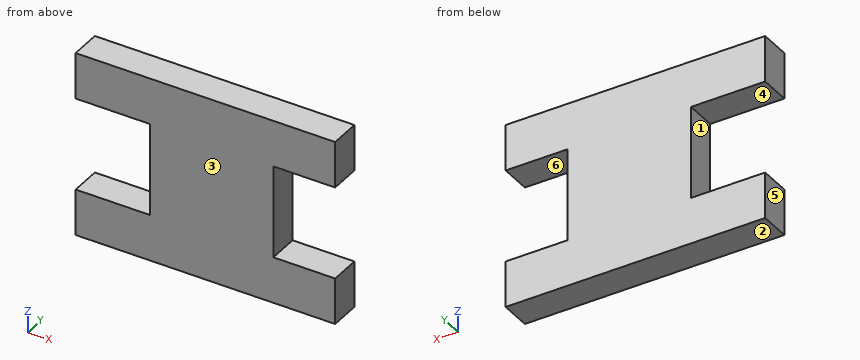
```python
from build123d import *

# Parameters (mm, degrees)
SKETCH1_W           = 95
SKETCH1_H           = 30
SKETCH1_R           = 7
SKETCH1_R_2         = 1
BOSS_EXTRUDE1_DEPTH = 5
SKETCH3_W           = 5
SKETCH3_H           = 10
CUT_EXTRUDE2_DEPTH  = 10
SKETCH4_R           = 7
SKETCH4_R_2         = 1
CUT_EXTRUDE3_DEPTH  = 10
FILLET1_R           = 10
CUT_EXTRUDE4_REACH  = 7
SKETCH5_R           = 2.05
BOSS_EXTRUDE2_DEPTH = 5
CUT_EXTRUDE5_DEPTH  = 5


with BuildPart() as part:
    # Sketch1 → Boss-Extrude1 (new body)
    with BuildSketch(Plane(origin=(0, 0, 0), x_dir=(1, 0, 0), z_dir=(0, 1, 0))):
        Rectangle(SKETCH1_W, SKETCH1_H)
        with Locations((-32.5, 0)):
            Circle(SKETCH1_R, mode=Mode.SUBTRACT)
        with Locations((-42.9, 0)):
            Circle(SKETCH1_R_2, mode=Mode.SUBTRACT)
        with Locations((-45.9, 0)):
            Circle(SKETCH1_R_2, mode=Mode.SUBTRACT)
        with Locations((-32.5, 10.4)):
            Circle(SKETCH1_R_2, mode=Mode.SUBTRACT)
        with Locations((-32.5, 13.4)):
            Circle(SKETCH1_R_2, mode=Mode.SUBTRACT)
        with Locations((-22.1, 0)):
            Circle(SKETCH1_R_2, mode=Mode.SUBTRACT)
        with Locations((-19.1, 0)):
            Circle(SKETCH1_R_2, mode=Mode.SUBTRACT)
        with Locations((-32.5, -10.4)):
            Circle(SKETCH1_R_2, mode=Mode.SUBTRACT)
        with Locations((-32.5, -13.4)):
            Circle(SKETCH1_R_2, mode=Mode.SUBTRACT)
    extrude(amount=BOSS_EXTRUDE1_DEPTH)

    # Sketch3 → Cut-Extrude2 (cut)
    with BuildSketch(Plane(origin=(0, 5, 0), x_dir=(1, 0, 0), z_dir=(0, 1, 0))):
        with Locations((-5, 0)):
            Rectangle(SKETCH3_W, SKETCH3_H)
    extrude(amount=-CUT_EXTRUDE2_DEPTH, mode=Mode.SUBTRACT)

    # Sketch4 → Cut-Extrude3 (cut)
    with BuildSketch(Plane(origin=(0, 5, 0), x_dir=(1, 0, 0), z_dir=(0, 1, 0))):
        with Locations((-32.5, 0)):
            Circle(SKETCH4_R)
        with Locations((-32.5, -13.4)):
            Circle(SKETCH4_R_2)
        with Locations((-32.5, -10.4)):
            Circle(SKETCH4_R_2)
        with Locations((-42.9, 0)):
            Circle(SKETCH4_R_2)
        with Locations((-45.9, 0)):
            Circle(SKETCH4_R_2)
        with Locations((-32.5, 13.4)):
            Circle(SKETCH4_R_2)
        with Locations((-22.1, 0)):
            Circle(SKETCH4_R_2)
        with Locations((-19.1, 0)):
            Circle(SKETCH4_R_2)
        with Locations((-32.5, 10.4)):
            Circle(SKETCH4_R_2)
        with Locations((27.5, -13.4)):
            Circle(SKETCH4_R_2)
        with Locations((27.5, -10.4)):
            Circle(SKETCH4_R_2)
        with Locations((40.9, 0)):
            Circle(SKETCH4_R_2)
        with Locations((37.9, 0)):
            Circle(SKETCH4_R_2)
        with Locations((27.5, 0)):
            Circle(SKETCH4_R)
        with Locations((27.5, 10.4)):
            Circle(SKETCH4_R_2)
        with Locations((27.5, 13.4)):
            Circle(SKETCH4_R_2)
        with Locations((17.1, 0)):
            Circle(SKETCH4_R_2)
        with Locations((14.1, 0)):
            Circle(SKETCH4_R_2)
    extrude(amount=-CUT_EXTRUDE3_DEPTH, mode=Mode.SUBTRACT)

    # Fillet1
    fillet1_edges = [part.edges().sort_by_distance(p)[0] for p in [
        (47.5, 2.5, 15),
        (-47.5, 2.5, 15),
        (-47.5, 2.5, -15),
        (47.5, 2.5, -15),
    ]]
    fillet(fillet1_edges, radius=FILLET1_R)

    # Sketch5 → Cut-Extrude4 (cut, up to next)
    with BuildSketch(Plane(origin=(0, 5, 0), x_dir=(1, 0, 0), z_dir=(0, 1, 0)), mode=Mode.PRIVATE) as cut_extrude4_sk1:
        with Locations((-7.5, 5)):
            Circle(SKETCH5_R)
    cut_extrude4_tool1 = extrude(cut_extrude4_sk1.sketch, amount=-CUT_EXTRUDE4_REACH, mode=Mode.PRIVATE) & part.part
    add(cut_extrude4_tool1.solids().sort_by_distance((-7.5, 5, -5))[0], mode=Mode.SUBTRACT)
    # Sketch5 → Cut-Extrude4 (cut, up to next)
    with BuildSketch(Plane(origin=(0, 5, 0), x_dir=(1, 0, 0), z_dir=(0, 1, 0)), mode=Mode.PRIVATE) as cut_extrude4_sk2:
        with Locations((-2.5, 5)):
            Circle(SKETCH5_R)
    cut_extrude4_tool2 = extrude(cut_extrude4_sk2.sketch, amount=-CUT_EXTRUDE4_REACH, mode=Mode.PRIVATE) & part.part
    add(cut_extrude4_tool2.solids().sort_by_distance((-2.5, 5, -5))[0], mode=Mode.SUBTRACT)
    # Sketch5 → Cut-Extrude4 (cut, up to next)
    with BuildSketch(Plane(origin=(0, 5, 0), x_dir=(1, 0, 0), z_dir=(0, 1, 0)), mode=Mode.PRIVATE) as cut_extrude4_sk3:
        with Locations((-2.5, -5)):
            Circle(SKETCH5_R)
    cut_extrude4_tool3 = extrude(cut_extrude4_sk3.sketch, amount=-CUT_EXTRUDE4_REACH, mode=Mode.PRIVATE) & part.part
    add(cut_extrude4_tool3.solids().sort_by_distance((-2.5, 5, 5))[0], mode=Mode.SUBTRACT)
    # Sketch5 → Cut-Extrude4 (cut, up to next)
    with BuildSketch(Plane(origin=(0, 5, 0), x_dir=(1, 0, 0), z_dir=(0, 1, 0)), mode=Mode.PRIVATE) as cut_extrude4_sk4:
        with Locations((-7.5, -5)):
            Circle(SKETCH5_R)
    cut_extrude4_tool4 = extrude(cut_extrude4_sk4.sketch, amount=-CUT_EXTRUDE4_REACH, mode=Mode.PRIVATE) & part.part
    add(cut_extrude4_tool4.solids().sort_by_distance((-7.5, 5, 5))[0], mode=Mode.SUBTRACT)

    # Sketch6 → Boss-Extrude2 (add)
    with BuildSketch(Plane(origin=(0, 5, 0), x_dir=(1, 0, 0), z_dir=(0, 1, 0))):
        Polygon((-22.5, 15), (19.5, 15), (19.5, 7.5), (9.5, 7.5), (9.5, -7.5), (19.5, -7.5), (19.5, -15), (-22.5, -15), (-22.5, -7.5), (-10.5, -7.5), (-10.5, 7.5), (-22.5, 7.5), align=None)
    extrude(amount=BOSS_EXTRUDE2_DEPTH)

    # Sketch8 → Cut-Extrude5 (cut)
    with BuildSketch(Plane.XZ):
        with BuildLine():
            Line((47.5, -5), (47.5, 5))
            ThreePointArc((47.5, 5), (44.571067812, 12.071067812), (37.5, 15))
            Line((37.5, 15), (-37.5, 15))
            ThreePointArc((-37.5, 15), (-44.571067812, 12.071067812), (-47.5, 5))
            Line((-47.5, 5), (-47.5, -5))
            ThreePointArc((-47.5, -5), (-44.571067812, -12.071067812), (-37.5, -15))
            Line((-37.5, -15), (37.5, -15))
            ThreePointArc((37.5, -15), (44.571067812, -12.071067812), (47.5, -5))
        make_face()
    extrude(amount=-CUT_EXTRUDE5_DEPTH, mode=Mode.SUBTRACT)


solid = part.part
```
Geometry check sheet. Reference: the model listing, model coordinates, mm. Face numbers are marked on the shaded views. A direction names the side the tool comes from. Coordinates: 2 decimals unless noted, no trailing zeros. Order: outer loops, then holes, each group sorted by start corner. A loop starts at its lowest first (then second) coordinate and runs counter-clockwise, first axis right, second up. Notation, with made-up numbers: (60, -11) - (78, -11) arc R19 cw to (78, -5) - close; hole circle Ø5 at (18.5, -29.75). An arc over 180 degrees is marked (long way). Answer as a JSON object with one key per item and string values. Group by question number.
Item 1: Sectioned sample at A-A, the plane x = 14. Record the cut outline in (y, z), and give its area (3 significant figures).
Item 2: Sectioned sample at C-C, the plane z = -6.5. Record the cut outline in (x, y).
Item 3: Draft check along Z on the marked faces 1, 2 and 3. Enter one of: +Z half, -Z half, draft (parallel to the pull), parting line (faces both ways), or undercut.
Item 4: Sectioned sample at B-B, the plane y = 7.65. Record the cut outline in (x, z), and give its area (3 significant figures).
Item 5: Scan lines: probe 1 along Z at (x, y) = (14.5, 9.15); probe 2 along X at (y, z) = (5.5, 6). Record each from-to range of solid material in increasing order.
Item 6: Tool access check on the marked faces 4, 5 and 6. Record the directions out of +Z, -Z, +X, -X, +Y, -Y that give a thin tool (end or side, any length) a straight path to the whole face; none if there is none.
Resolved:
{
 "1": {"outline": "(5, -15) - (10, -15) - (10, -7.5) - (5, -7.5) - close; (5, 7.5) - (10, 7.5) - (10, 15) - (5, 15) - close", "area": "75.0 mm^2"},
 "2": {"outline": "(-10.5, 5) - (9.5, 5) - (9.5, 10) - (-10.5, 10) - close"},
 "3": {"face 1": "undercut", "face 2": "-Z half", "face 3": "draft"},
 "4": {"outline": "(-22.5, -15) - (19.5, -15) - (19.5, -7.5) - (9.5, -7.5) - (9.5, 7.5) - (19.5, 7.5) - (19.5, 15) - (-22.5, 15) - (-22.5, 7.5) - (-10.5, 7.5) - (-10.5, -7.5) - (-22.5, -7.5) - close", "area": "930 mm^2"},
 "5": {"probe 1": "-15 to -7.5, 7.5 to 15", "probe 2": "-10.5 to 9.5"},
 "6": {"face 4": "-X, +Y, -Y", "face 5": "+Z, -Z, -X, +Y, -Y", "face 6": "+X, +Y, -Y"}
}
